```python
from build123d import *

# Parameters (mm, degrees)
EXTRUDE_THIN1_DEPTH               = 533.4
F_3_16_0_1875_DIAMETER_HOLE1_D    = 4.7625
F_3_16_0_195_DIAMETER_HOLE1_D     = 4.953
F_3_16_0_195_DIAMETER_HOLE1_DEPTH = 1.5875


with BuildPart() as part:
    # Sketch1 → Extrude-Thin1 (new body)
    with BuildSketch(Plane.XY):
        with BuildLine():
            Line((-12.7, 19.05), (-12.7, -19.05))
            ThreePointArc((-12.7, -19.05), (-10.840128061, -23.540128061), (-6.35, -25.4))
            Line((-6.35, -25.4), (6.35, -25.4))
            ThreePointArc((6.35, -25.4), (10.840128061, -23.540128061), (12.7, -19.05))
            Line((12.7, -19.05), (12.7, 19.05))
            ThreePointArc((12.7, 19.05), (10.840128061, 23.540128061), (6.35, 25.4))
            Line((6.35, 25.4), (-6.35, 25.4))
            ThreePointArc((-6.35, 25.4), (-10.840128061, 23.540128061), (-12.7, 19.05))
        make_face()
        with BuildLine():
            Line((-11.1125, 19.05), (-11.1125, -19.05))
            ThreePointArc((-11.1125, -19.05), (-9.717596045, -22.417596045), (-6.35, -23.8125))
            Line((-6.35, -23.8125), (6.35, -23.8125))
            ThreePointArc((6.35, -23.8125), (9.717596045, -22.417596045), (11.1125, -19.05))
            Line((11.1125, -19.05), (11.1125, 19.05))
            ThreePointArc((11.1125, 19.05), (9.717596045, 22.417596045), (6.35, 23.8125))
            Line((6.35, 23.8125), (-6.35, 23.8125))
            ThreePointArc((-6.35, 23.8125), (-9.717596045, 22.417596045), (-11.1125, 19.05))
        make_face(mode=Mode.SUBTRACT)
    extrude(amount=EXTRUDE_THIN1_DEPTH)

    # 3/16 (0.1875) Diameter Hole1 (through all)
    with Locations(Plane(origin=(0, 25.4, 527.05), x_dir=(0, 0, 1), z_dir=(0, 1, 0))):
        with Locations((0, 0), (-520.7, 0), (-495.3, 0), (-469.9, 0), (-25.4, 0), (-50.8, 0)):
            Hole(F_3_16_0_1875_DIAMETER_HOLE1_D / 2)

    # 3/16 (0.195) Diameter Hole1
    with Locations(Plane(origin=(0, -25.4, 0), x_dir=(-1, 0, 0), z_dir=(0, -1, 0))):
        with Locations((-6.331002809, -114.316339601), (0.281657017, -139.649227909), (-5.805002341, -165.113616334), (0.807657485, -190.446504642), (-3.175, -419.1), (2.911659358, -393.635611575), (-3.701000468, -368.302723267), (2.385658889, -342.838334842)):
            Hole(F_3_16_0_195_DIAMETER_HOLE1_D / 2, depth=F_3_16_0_195_DIAMETER_HOLE1_DEPTH)


solid = part.part
```
CAD build for the part. Positions are in the model's coordinates, mm. A direction names the side the tool comes from. Coordinates: 2 decimals unless noted, no trailing zeros. Order: outer loops, then holes, each group sorted by start corner. A loop starts at its lowest first (then second) coordinate and runs counter-clockwise, first axis right, second up. Notation, with made-up numbers: (66, 79) - (90, 79) arc R14 cw to (90, 95) - close; hole circle Ø7 at (76.5, 74). An arc over 180 degrees is marked (long way). Use a Markdown table: item, result. Add a question column.
(1) Drill centre lines: line 1 along X through (y, z) = (-11.5, 90.5); line 2 along Y through (x, z) = (-7, 218); line 3 along Y through (x, z) = (-8, 337.5). Where is each one in solid material? Low to high. Write a range as [from, to].
(2) Pull direction Y, two halves, no side cores. Call faces 1 (the face through (0, -25.4, 263)), 2 (the face through (-12.7, 0, 263)), 3 (the face through (11.112, 0, 263)), 4 (the face through (0, -23.812, 263)): +Y half, -Y half, draft (parallel to the pull), parting line (faces both ways), or undercut.
(3) Flat gauge pins, fed straight in: pin 1 (3 mm diameter, centred on x = 0, z = 31.75, fed in from -Y); pin 2 (2 mm diameter, centred on x = 8, z = 115.5, fed in from -Y); pin 3 (3 mm diameter, centred on x = 3.7, z = 368.3, fed in from -Y); pin 4 (3 mm diameter, centred on x = -8, z = 62, fed in from +Y). Where does each tip first touch, or does it go through?
(4) Which spindle directions (+Z, -Z, +X, -X, +Y, -Y) get a long thin tool onto all of the face, cutting with end or side? Do faces 5 (the face through (12.7, 0, 263)), 6 (the face through (-11.112, 0, 263)). Say none if no direction does.
(5) Saw through at A-A (y = -1.5). Give the cut face in (x, z), then the cut area to 3 significant figures.
Solved:
| question | item | result |
|---|---|---|
| 1 | line 1 | x = [-12.7, -11.11], [11.11, 12.7] |
| 1 | line 2 | y = [-25.37, -23.77], [23.77, 25.37] |
| 1 | line 3 | y = [-25.18, -23.52], [23.52, 25.18] |
| 2 | face 1 | -Y half |
| 2 | face 2 | draft |
| 2 | face 3 | undercut |
| 2 | face 4 | undercut |
| 3 | pin 1 | passes through |
| 3 | pin 2 | stops at y = -25.27 |
| 3 | pin 3 | stops at y = 23.81 |
| 3 | pin 4 | stops at y = 25.4 |
| 4 | face 5 | +Z, -Z, +X, +Y, -Y |
| 4 | face 6 | +Z, -Z |
| 5 | outline | (-12.7, 0) - (-11.11, 0) - (-11.11, 533.4) - (-12.7, 533.4) - close; (11.11, 0) - (12.7, 0) - (12.7, 533.4) - (11.11, 533.4) - close |
| 5 | area | 1,690 mm² |
